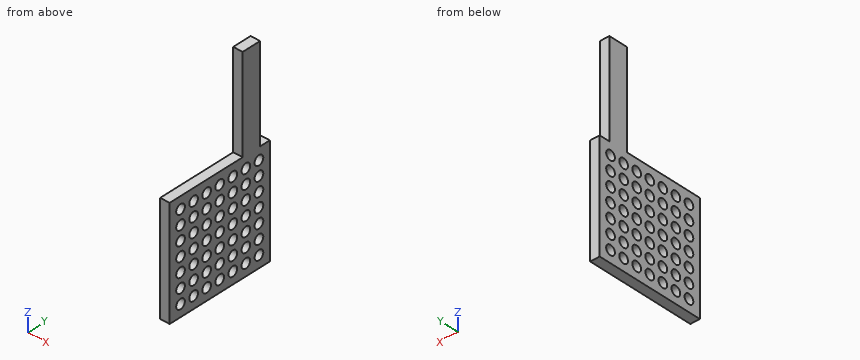
```python
from build123d import *

# Parameters (mm, degrees)
F0_R     = 0.5
F1_DEPTH = 1


# Not quite as in the source:
# - a feature names something its author has since deleted; it is built from what else it names


with BuildPart() as f1:
    # F0 (on Right) → F1 (new body)
    with BuildSketch(Plane.YZ):
        Polygon((8.384144865, 0), (0, 0), (0, -11.5), (11.5, -11.5), (11.5, 0), (10.384144865, 0), (10.384144865, 10), (8.384144865, 10), align=None)
        with Locations((1.25, -10.249999141)):
            Circle(F0_R, mode=Mode.SUBTRACT)
        with Locations((2.75, -10.249999141)):
            Circle(F0_R, mode=Mode.SUBTRACT)
        with Locations((1.25, -8.7499995705)):
            Circle(F0_R, mode=Mode.SUBTRACT)
        with Locations((1.25, -7.25)):
            Circle(F0_R, mode=Mode.SUBTRACT)
        with Locations((2.75, -8.7499995705)):
            Circle(F0_R, mode=Mode.SUBTRACT)
        with Locations((2.75, -7.25)):
            Circle(F0_R, mode=Mode.SUBTRACT)
        with Locations((4.25, -10.249999141)):
            Circle(F0_R, mode=Mode.SUBTRACT)
        with Locations((4.25, -8.7499995705)):
            Circle(F0_R, mode=Mode.SUBTRACT)
        with Locations((4.25, -7.25)):
            Circle(F0_R, mode=Mode.SUBTRACT)
        with Locations((5.7488648942, -8.7499995705)):
            Circle(F0_R, mode=Mode.SUBTRACT)
        with Locations((1.25, -5.75)):
            Circle(F0_R, mode=Mode.SUBTRACT)
        with Locations((1.25, -4.25)):
            Circle(F0_R, mode=Mode.SUBTRACT)
        with Locations((2.75, -5.75)):
            Circle(F0_R, mode=Mode.SUBTRACT)
        with Locations((2.75, -4.25)):
            Circle(F0_R, mode=Mode.SUBTRACT)
        with Locations((1.25, -2.7500004295)):
            Circle(F0_R, mode=Mode.SUBTRACT)
        with Locations((1.25, -1.250000859)):
            Circle(F0_R, mode=Mode.SUBTRACT)
        with Locations((2.75, -2.7500004295)):
            Circle(F0_R, mode=Mode.SUBTRACT)
        with Locations((2.75, -1.250000859)):
            Circle(F0_R, mode=Mode.SUBTRACT)
        with Locations((4.25, -5.75)):
            Circle(F0_R, mode=Mode.SUBTRACT)
        with Locations((4.25, -4.25)):
            Circle(F0_R, mode=Mode.SUBTRACT)
        with Locations((4.25, -2.7500004295)):
            Circle(F0_R, mode=Mode.SUBTRACT)
        with Locations((4.25, -1.250000859)):
            Circle(F0_R, mode=Mode.SUBTRACT)
        with Locations((5.7488648942, -2.7500004295)):
            Circle(F0_R, mode=Mode.SUBTRACT)
        with Locations((5.75, -10.249999141)):
            Circle(F0_R, mode=Mode.SUBTRACT)
        with Locations((7.25, -10.249999141)):
            Circle(F0_R, mode=Mode.SUBTRACT)
        with Locations((5.75, -7.25)):
            Circle(F0_R, mode=Mode.SUBTRACT)
        with Locations((7.25, -8.7499995705)):
            Circle(F0_R, mode=Mode.SUBTRACT)
        with Locations((7.25, -7.25)):
            Circle(F0_R, mode=Mode.SUBTRACT)
        with Locations((8.75, -10.249999141)):
            Circle(F0_R, mode=Mode.SUBTRACT)
        with Locations((10.25, -10.249999141)):
            Circle(F0_R, mode=Mode.SUBTRACT)
        with Locations((8.75, -8.7499995705)):
            Circle(F0_R, mode=Mode.SUBTRACT)
        with Locations((8.75, -7.25)):
            Circle(F0_R, mode=Mode.SUBTRACT)
        with Locations((10.25, -8.7499995705)):
            Circle(F0_R, mode=Mode.SUBTRACT)
        with Locations((10.25, -7.25)):
            Circle(F0_R, mode=Mode.SUBTRACT)
        with Locations((5.75, -5.75)):
            Circle(F0_R, mode=Mode.SUBTRACT)
        with Locations((5.75, -4.25)):
            Circle(F0_R, mode=Mode.SUBTRACT)
        with Locations((7.25, -5.75)):
            Circle(F0_R, mode=Mode.SUBTRACT)
        with Locations((7.25, -4.25)):
            Circle(F0_R, mode=Mode.SUBTRACT)
        with Locations((5.75, -1.250000859)):
            Circle(F0_R, mode=Mode.SUBTRACT)
        with Locations((7.25, -2.7500004295)):
            Circle(F0_R, mode=Mode.SUBTRACT)
        with Locations((7.25, -1.250000859)):
            Circle(F0_R, mode=Mode.SUBTRACT)
        with Locations((8.75, -5.75)):
            Circle(F0_R, mode=Mode.SUBTRACT)
        with Locations((8.75, -4.25)):
            Circle(F0_R, mode=Mode.SUBTRACT)
        with Locations((10.25, -5.75)):
            Circle(F0_R, mode=Mode.SUBTRACT)
        with Locations((10.25, -4.25)):
            Circle(F0_R, mode=Mode.SUBTRACT)
        with Locations((8.75, -2.7500004295)):
            Circle(F0_R, mode=Mode.SUBTRACT)
        with Locations((8.75, -1.250000859)):
            Circle(F0_R, mode=Mode.SUBTRACT)
        with Locations((10.25, -2.7500004295)):
            Circle(F0_R, mode=Mode.SUBTRACT)
        with Locations((10.25, -1.250000859)):
            Circle(F0_R, mode=Mode.SUBTRACT)
    extrude(amount=F1_DEPTH)


solid = f1.part
```
Design review of the part built by this model. Coordinates are the model's own, in mm. Round coordinates to 2 decimals unless told otherwise and drop trailing zeros. Write each loop counter-clockwise with the first axis right and the second up, starting at its lowest first coordinate (ties: lowest second). Pieces come first, ordered by that corner, then holes. Notation, with made-up numbers: (-20.75, 21.25) -> (12.25, 21.25) arc R14 ccw to (12.25, 45.25) -> close; hole circle Ø8 at (52, 21). An arc over 180 degrees is marked (long way). Answer in a Markdown table with one row per item.
Q1. Take a section at D-D, the plane y = 3.5. State the section outline as (x, z) points, then the cut area to 3 significant figures.
The answers:
| item | result |
|---|---|
| outline | (0, -11.5) -> (1, -11.5) -> (1, 0) -> (0, 0) -> close |
| area | 11.5 mm² |
Q2. To check wall thickness, follow L1, parallel to Y at x = 0.2, z = 8.75; L2, parallel to Z at x = 0.55, y = 5. State the ranges of each line that lie inside material, in increasing order. Write a range as [from, to].
The answers:
| item | result |
|---|---|
| L1 | [8.38, 10.38] |
| L2 | [-11.5, 0] |
Q3. Take a section at A-A, the plane y = 8.75. Count the separate pieces of the cut face and the enclosed holes in it, then the cut area to 3 significant figures.
The answers:
| item | result |
|---|---|
| separate pieces | 8 |
| enclosed holes | 0 |
| area | 14.5 mm² |
Q4. Clearance check with a flat-ended pin moving along its axis: pin 1 Ø0.5 at (x, y) = (0.5, 6) entering from +Z. State where the tip first meets the part, or that it passes through.
The answers:
| item | result |
|---|---|
| pin 1 | z = 0 |
